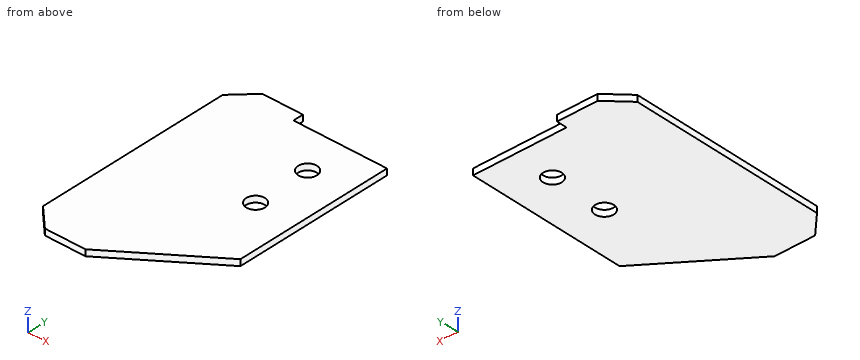
Autodesk Fusion 360 part; units mm, degrees
sketch "スケッチ1" plane through (0, 0, 0) normal (0, 0, 1) x (1, 0, 0)
  line L0 (-15.5, 115) -> (-74.5, 115)
  line L1 (-74.5, 115) -> (-74.5, -115)
  line L2 (-74.5, -115) -> (-15.5, -115)
  line L3 (74.5, -50) -> (74.5, 105)
  line L4 (68.0217, 105) -> (-74.5, -115) construction
  line L5 (-74.5, 115) -> (45.8131, -70.7183) construction
  line L6 (-15.5, 115) -> (-15.5, 105)
  line L7 (-15.5, 105) -> (74.5, 105)
  line L8 (-74.5, -115) -> (-15.5, -115) construction
  line L9 (74.5, -50) -> (-15.5, -115)
  dimension "d2" = 230
  dimension "d5" = 59
extrude "押し出し1" add sketch "スケッチ1" along normal blind 6
chamfer "面取り1" distance 20 angle 45 2 edges at (-74.5, -115, 3) (-74.5, 115, 3)
sketch "スケッチ2" plane through (0, 0, 6) normal (0, 0, 1) x (-1, 0, 0)
  line L0 (54.5, -115) -> (74.5, -95)
  line L1 (74.5, -95) -> (74.5, 95)
  line L2 (74.5, 95) -> (54.5, 115)
  line L3 (54.5, 115) -> (15.5, 115)
  line L4 (15.5, 115) -> (-74.5, 50)
  line L5 (-74.5, 50) -> (-74.5, -105)
  line L6 (-74.5, -105) -> (15.5, -105)
  line L7 (15.5, -105) -> (15.5, -115)
  line L8 (15.5, -115) -> (54.5, -115)
  line L9 (-74.5, -105) -> (-34.5, -105) construction
  line L10 (-34.5, -105) -> (-34.5, -65) construction
  line L11 (-34.5, -65) -> (-74.5, -65) construction
  line L12 (-74.5, -65) -> (-74.5, -105) construction
  line L13 (-34.5, -65) -> (-34.5, -10) construction
  point P0 (-34.5, -65)
  point P1 (-34.5, -10)
  dimension "d10" = 40
  dimension "d11" = 40
  dimension "d12" = 55
hole "穴1" at (34.5, 65, 6) at (34.5, 10, 6) direction (0, 0, -1) diameter 18 end through all
equation "d5 = 20 mm + 39 mm"
Build history of the part. All positions in model axes, mm. Coordinates: 2 decimals unless noted, no trailing zeros. Order: outer loops, then holes, each group sorted by start corner. A loop starts at its lowest first (then second) coordinate and runs counter-clockwise, first axis right, second up. Notation, with made-up numbers: (53.5, 52) -> (86.5, 52) arc R30 cw to (86.5, 81) -> close; hole circle Ø1 at (83.25, 39.5). An arc over 180 degrees is marked (long way). Answer in a Markdown table with one row per item. Add a question column.
Q1. Band-saw the part on A-A, the plane z = 1.35. List the corners of the cut face in (x, y).
Q2. Drop a flat-ended pin along its axis: pin 1 (1 mm diameter, centred on x = 33.5, z = 5, fed in from +Y). Give the stop position or say it passes through.
Q3. Wall check: line 1 along X through (y, z) = (10, 3.9); line 2 along Y through (x, z) = (27.5, 2.65); line 3 along Y through (x, z) = (34.5, 3.1). Give the ranges that are in metal, low to high. Write a range as [from, to].
Q4. Band-saw the part on C-C, the plane x = 34.5. List the corners of the cut face in (y, z).
Q5. Band-saw the part on B-B, the plane y = 10. List the corners of the cut face in (x, z).
Q6. Band-saw the part on D-D, the plane y = -59. List the corners of the cut face in (x, z), then the cut area to 3 significant figures.
Answers follow:
| question | item | result |
|---|---|---|
| 1 | outline | (-74.5, -95) -> (-54.5, -115) -> (-15.5, -115) -> (74.5, -50) -> (74.5, 105) -> (-15.5, 105) -> (-15.5, 115) -> (-54.5, 115) -> (-74.5, 95) -> close; hole circle Ø18 at (34.5, 10); hole circle Ø18 at (34.5, 65) |
| 2 | pin 1 | y = 105 |
| 3 | line 1 | [-74.5, 25.5], [43.5, 74.5] |
| 3 | line 2 | [-83.94, 4.34], [15.66, 59.34], [70.66, 105] |
| 3 | line 3 | [-78.89, 1], [19, 56], [74, 105] |
| 4 | outline | (-78.89, 0) -> (1, 0) -> (1, 6) -> (-78.89, 6) -> close; (19, 0) -> (56, 0) -> (56, 6) -> (19, 6) -> close; (74, 0) -> (105, 0) -> (105, 6) -> (74, 6) -> close |
| 5 | outline | (-74.5, 0) -> (25.5, 0) -> (25.5, 6) -> (-74.5, 6) -> close; (43.5, 0) -> (74.5, 0) -> (74.5, 6) -> (43.5, 6) -> close |
| 6 | outline | (-74.5, 0) -> (62.04, 0) -> (62.04, 6) -> (-74.5, 6) -> close |
| 6 | area | 819 mm^2 |
